Could you check a few things on this model? Use its own coordinates, in mm. A direction names the side the tool comes from. Coordinates: 2 decimals unless noted, no trailing zeros. Loops run counter-clockwise (first coordinate to the right, second up) from the corner with the lowest first, then second, coordinate; pieces in that order, holes last. Notation, with made-up numbers: (71.5, 14.25) -> (121.5, 14.25) arc R15 cw to (121.5, 25.25) -> close; hole circle Ø5 at (88, 30). An arc over 180 degrees is marked (long way). One line per question, with ' | ' between items. Start each with the question number.
(1) Suppose I cut it at D-D (x = -37). Please give me the cut outline in (y, z).
(2) Suppose I cut it at C-C (z = 26). Please give me the cut outline in (x, y), plus the area to 3 significant figures.
(3) Which directions (+Z, -Z, +X, -X, +Y, -Y) give clear straight access to the entire face, cutting with the end or side of a thin tool? Please do faces 4 (the face through (-43, 44, 0)), 5 (the face through (-5.5, 82, 31)).
(4) Suppose I cut it at A-A (y = 21.5). Please give me the cut outline in (x, z).
(5) If I drill on line 1 along X through (y, z) = (2, 19.5); line 2 along Y through (x, z) = (-60.5, 12); line 3 along Z through (x, y) = (-52.5, 44), over which ranges is the centre line in solid material (lowest first)?
(6) I'm going to push flat-ended pins straight in: pin 1 Ø9 at (y, z) = (81.5, 23.5) entering from +X; pin 2 Ø4 at (x, z) = (-40.5, 22.5) entering from +Y. Where does each tip first touch, or does it pass through?
(7) Suppose I cut it at B-B (z = 37.5). Please give me the cut outline in (x, y), plus the area to 3 significant figures.
(8) If we mould it in two halves opening along Y, with no side actions, what happens to faces 1 (the face through (-9, 78, 31)), 2 (the face through (-61.042, -1.479, 40.815)), 3 (the face through (-43, -3, 25))? For each: pulls with the +Y half, pulls with the -Y half, needs draft (parallel to the pull), parting line crosses it, or undercut.
```python
from build123d import *

# Parameters (mm, degrees)
SKETCH1_W           = 85
SKETCH1_H           = 50
BOSS_EXTRUDE1_DEPTH = 90
CUT_EXTRUDE1_REACH  = 135.51
SKETCH2_W           = 62
SKETCH2_H           = 40
SKETCH3_W           = 85
SKETCH3_H           = 16
BOSS_EXTRUDE2_DEPTH = 24
CUT_EXTRUDE2_REACH  = 130.378
SKETCH4_W           = 6
SKETCH4_H           = 8
SKETCH5_W           = 85
SKETCH5_H           = 50
BOSS_EXTRUDE3_DEPTH = 3
CUT_EXTRUDE3_REACH  = 135.51
SKETCH6_R           = 3
CHAMFER1_SIZE       = 4


with BuildPart() as part:
    # Sketch1 → Boss-Extrude1 (new body)
    with BuildSketch(Plane(origin=(0, 0, 0), x_dir=(1, 0, 0), z_dir=(0, 1, 0))):
        with Locations((-42.5, -25)):
            Rectangle(SKETCH1_W, SKETCH1_H)
    extrude(amount=BOSS_EXTRUDE1_DEPTH)

    # Sketch2 → Cut-Extrude1 (cut, up to next)
    with BuildSketch(Plane(origin=(0, 90, 0), x_dir=(1, 0, 0), z_dir=(0, 1, 0)), mode=Mode.PRIVATE) as cut_extrude1_sk1:
        with Locations((-42.5, -30)):
            Rectangle(SKETCH2_W, SKETCH2_H)
    cut_extrude1_tool1 = extrude(cut_extrude1_sk1.sketch, amount=-CUT_EXTRUDE1_REACH, mode=Mode.PRIVATE) & part.part
    add(cut_extrude1_tool1.solids().sort_by_distance((-42.5, 90, 30))[0], mode=Mode.SUBTRACT)

    # Sketch3 → Boss-Extrude2 (add)
    with BuildSketch(Plane(origin=(0, 90, 0), x_dir=(1, 0, 0), z_dir=(0, 1, 0))):
        with Locations((-42.5, -8)):
            Rectangle(SKETCH3_W, SKETCH3_H)
    extrude(amount=-BOSS_EXTRUDE2_DEPTH)

    # Sketch4 → Cut-Extrude2 (cut, up to next)
    with BuildSketch(Plane.XY.offset(16), mode=Mode.PRIVATE) as cut_extrude2_sk1:
        with Locations((-76.5, 82)):
            Rectangle(SKETCH4_W, SKETCH4_H)
    cut_extrude2_tool1 = extrude(cut_extrude2_sk1.sketch, amount=CUT_EXTRUDE2_REACH, mode=Mode.PRIVATE) & part.part
    # Sketch4 → Cut-Extrude2 (cut, up to next)
    with BuildSketch(Plane.XY.offset(16), mode=Mode.PRIVATE) as cut_extrude2_sk2:
        with Locations((-8.5, 82)):
            Rectangle(SKETCH4_W, SKETCH4_H)
    cut_extrude2_tool2 = extrude(cut_extrude2_sk2.sketch, amount=CUT_EXTRUDE2_REACH, mode=Mode.PRIVATE) & part.part
    add(cut_extrude2_tool1.solids().sort_by_distance((-76.5, 82, 16))[0], mode=Mode.SUBTRACT)
    add(cut_extrude2_tool2.solids().sort_by_distance((-8.5, 82, 16))[0], mode=Mode.SUBTRACT)

    # Sketch5 → Boss-Extrude3 (add)
    with BuildSketch(Plane.XZ):
        with Locations((-42.5, 25)):
            Rectangle(SKETCH5_W, SKETCH5_H)
    extrude(amount=BOSS_EXTRUDE3_DEPTH)

    # Sketch6 → Cut-Extrude3 (cut, up to next)
    with BuildSketch(Plane(origin=(0, 0, 0), x_dir=(1, 0, 0), z_dir=(0, 1, 0)), mode=Mode.PRIVATE) as cut_extrude3_sk1:
        with Locations(Location((-63.406474548, -19.640219105, 0), (0, 0, 270))):
            Circle(SKETCH6_R)
    cut_extrude3_tool1 = extrude(cut_extrude3_sk1.sketch, amount=-CUT_EXTRUDE3_REACH, mode=Mode.PRIVATE) & part.part
    # Sketch6 → Cut-Extrude3 (cut, up to next)
    with BuildSketch(Plane(origin=(0, 0, 0), x_dir=(1, 0, 0), z_dir=(0, 1, 0)), mode=Mode.PRIVATE) as cut_extrude3_sk2:
        with Locations(Location((-20.861133032, -19.640219105, 0), (0, 0, 270))):
            Circle(SKETCH6_R)
    cut_extrude3_tool2 = extrude(cut_extrude3_sk2.sketch, amount=-CUT_EXTRUDE3_REACH, mode=Mode.PRIVATE) & part.part
    # Sketch6 → Cut-Extrude3 (cut, up to next)
    with BuildSketch(Plane(origin=(0, 0, 0), x_dir=(1, 0, 0), z_dir=(0, 1, 0)), mode=Mode.PRIVATE) as cut_extrude3_sk3:
        with Locations(Location((-20.861133032, -39.202410137, 0), (0, 0, 270))):
            Circle(SKETCH6_R)
    cut_extrude3_tool3 = extrude(cut_extrude3_sk3.sketch, amount=-CUT_EXTRUDE3_REACH, mode=Mode.PRIVATE) & part.part
    # Sketch6 → Cut-Extrude3 (cut, up to next)
    with BuildSketch(Plane(origin=(0, 0, 0), x_dir=(1, 0, 0), z_dir=(0, 1, 0)), mode=Mode.PRIVATE) as cut_extrude3_sk4:
        with Locations(Location((-63.571834409, -39.202410137, 0), (0, 0, 270))):
            Circle(SKETCH6_R)
    cut_extrude3_tool4 = extrude(cut_extrude3_sk4.sketch, amount=-CUT_EXTRUDE3_REACH, mode=Mode.PRIVATE) & part.part
    add(cut_extrude3_tool1.solids().sort_by_distance((-63.406475, 0, 19.640219))[0], mode=Mode.SUBTRACT)
    add(cut_extrude3_tool2.solids().sort_by_distance((-20.861133, 0, 19.640219))[0], mode=Mode.SUBTRACT)
    add(cut_extrude3_tool3.solids().sort_by_distance((-20.861133, 0, 39.20241))[0], mode=Mode.SUBTRACT)
    add(cut_extrude3_tool4.solids().sort_by_distance((-63.571834, 0, 39.20241))[0], mode=Mode.SUBTRACT)

    # Chamfer1
    chamfer1_edges = [part.edges().sort_by_distance(p)[0] for p in [
        (-76.5, 86, 50),
        (-79.5, 82, 50),
        (-76.5, 78, 50),
        (-8.5, 78, 50),
        (-5.5, 82, 50),
        (-8.5, 86, 50),
    ]]
    chamfer(chamfer1_edges, length=CHAMFER1_SIZE - 0.0001)  # a hair under: the kernel refuses the full size


solid = part.part
```
Checks:
1) outline: (-3, 0) -> (90, 0) -> (90, 16) -> (66, 16) -> (66, 10) -> (0, 10) -> (0, 50) -> (-3, 50) -> close
2) outline: (-85, -3) -> (0, -3) -> (0, 90) -> (-11.5, 90) -> (-11.5, 86) -> (-5.5, 86) -> (-5.5, 78) -> (-11.5, 78) -> (-11.5, 0) -> (-73.5, 0) -> (-73.5, 78) -> (-79.5, 78) -> (-79.5, 86) -> (-73.5, 86) -> (-73.5, 90) -> (-85, 90) -> close | area: 2,230 mm^2
3) face 4: -Z, +X, -X, +Y, -Y | face 5: +Z
4) outline: (-85, 0) -> (0, 0) -> (0, 50) -> (-11.5, 50) -> (-11.5, 10) -> (-73.5, 10) -> (-73.5, 50) -> (-85, 50) -> close
5) line 1: x = -85 to -73.5, -11.5 to 0 | line 2: y = -3 to 0, 66 to 90 | line 3: z = 0 to 10
6) pin 1: stops at x = 0 | pin 2: stops at y = 0
7) outline: (-85, -3) -> (-66.04, -3) -> (-66.04, 0) -> (-73.5, 0) -> (-73.5, 78) -> (-79.5, 78) -> (-79.5, 86) -> (-73.5, 86) -> (-73.5, 90) -> (-85, 90) -> close; (-61.1, -3) -> (-23.33, -3) -> (-23.33, 0) -> (-61.1, 0) -> close; (-18.39, -3) -> (0, -3) -> (0, 90) -> (-11.5, 90) -> (-11.5, 86) -> (-5.5, 86) -> (-5.5, 78) -> (-11.5, 78) -> (-11.5, 0) -> (-18.39, 0) -> close | area: 2,200 mm^2
8) face 1: undercut | face 2: needs draft | face 3: pulls with the -Y half
